Geometry: final body of the model. Coordinates: model frame, mm. A direction names the side the tool comes from. Give positions to 0.01 mm unless a question says otherwise; leave off trailing zeros. Order: outer loops, then holes, each group sorted by start corner. A loop starts at its lowest first (then second) coordinate and runs counter-clockwise, first axis right, second up. Notation, with made-up numbers: M 30,35.5 L 87,35.5 A29 ccw 87,73.5 Z; hole C -13.5,29.25 d5. An arc over 180 degrees is marked long. Use CSV: the item, a comma, the result in double quotes.
```python
from build123d import *

# Parameters (mm, degrees)
SKETCH1_W           = 63.5
SKETCH1_H           = 19.05
BOSS_EXTRUDE1_DEPTH = 6.35
SKETCH2_R           = 2.0955
CUT_EXTRUDE1_DEPTH  = 34.750712955
SKETCH3_W           = 12.7
SKETCH3_H           = 6.35
CUT_EXTRUDE2_DEPTH  = 34.750712955
SKETCH4_W           = 47.625
SKETCH4_H           = 19.05
BOSS_EXTRUDE2_DEPTH = 6.35
SKETCH5_R           = 1.5875
CUT_EXTRUDE3_DEPTH  = 44.184668865
SKETCH6_R           = 1.5875
CUT_EXTRUDE4_DEPTH  = 44.184668865
FILLET3_R           = 6.35
FILLET4_R           = 2.54


with BuildPart() as part:
    # Sketch1 → Boss-Extrude1 (new body)
    with BuildSketch(Plane.XY):
        Rectangle(SKETCH1_W, SKETCH1_H)
    extrude(amount=BOSS_EXTRUDE1_DEPTH)

    # Sketch2 → Cut-Extrude1 (cut, through all)
    with BuildSketch(Plane.XY.offset(6.35)):
        Circle(SKETCH2_R)
    extrude(amount=-CUT_EXTRUDE1_DEPTH, mode=Mode.SUBTRACT)

    # Sketch3 → Cut-Extrude2 (cut, through all)
    with BuildSketch(Plane.XY.offset(6.35)):
        with Locations((-19.05, 0)):
            Rectangle(SKETCH3_W, SKETCH3_H)
    cut_extrude2 = extrude(amount=-CUT_EXTRUDE2_DEPTH, mode=Mode.SUBTRACT)

    # Mirror1: Cut-Extrude2 across plane
    add(cut_extrude2.mirror(Plane(origin=(0, 0, 0), x_dir=(0, 0, 1), z_dir=(1, 0, 0))), mode=Mode.SUBTRACT)

    # Sketch4 → Boss-Extrude2 (add)
    with BuildSketch(Plane.XY.offset(6.35)):
        with Locations((0, 19.05)):
            Rectangle(SKETCH4_W, SKETCH4_H)
    extrude(amount=-BOSS_EXTRUDE2_DEPTH)

    # Sketch5 → Cut-Extrude3 (cut, through all)
    with BuildSketch(Plane.XY.offset(6.35)):
        with Locations((-18.288, 19.05)):
            Circle(SKETCH5_R)
    cut_extrude3 = extrude(amount=-CUT_EXTRUDE3_DEPTH, mode=Mode.SUBTRACT)

    # Mirror2: Cut-Extrude3 across plane
    add(cut_extrude3.mirror(Plane(origin=(0, 0, 0), x_dir=(0, 0, 1), z_dir=(1, 0, 0))), mode=Mode.SUBTRACT)

    # Sketch6 → Cut-Extrude4 (cut, through all)
    with BuildSketch(Plane.XY.offset(6.35)):
        with Locations((0, 6.35)):
            Circle(SKETCH6_R)
    extrude(amount=-CUT_EXTRUDE4_DEPTH, mode=Mode.SUBTRACT)

    # Fillet3
    fillet3_edges = [part.edges().sort_by_distance(p)[0] for p in [
        (23.8125, 28.575, 3.175),
        (-23.8125, 28.575, 3.175),
        (31.75, -9.525, 3.175),
        (-31.75, -9.525, 3.175),
        (-31.75, 9.525, 3.175),
        (31.75, 9.525, 3.175),
    ]]
    fillet(fillet3_edges, radius=FILLET3_R)

    # Fillet4
    fillet4_edges = [part.edges().sort_by_distance(p)[0] for p in [
        (23.8125, 9.525, 3.175),
        (-23.8125, 9.525, 3.175),
    ]]
    fillet(fillet4_edges, radius=FILLET4_R)


solid = part.part
```
1. Section D-D, the plane y = 6.35. Return the cut outline in (x, z).
Answer:
outline,"M -30.9,0 L -1.59,0 L -1.59,6.35 L -30.9,6.35 Z; M 1.59,0 L 30.9,0 L 30.9,6.35 L 1.59,6.35 Z"
2. Pull-direction query (Y, two-part tool) for faces 1 (the face through (0, 28.575, 3)), 2 (the face through (-12.7, 0, 3)), 3 (the face through (0, 10, 6.35)); classes: +Y half, -Y half, draft (parallel to the pull), parting line (faces both ways), or undercut.
Answer:
face 1,"+Y half"
face 2,"undercut"
face 3,"draft"
3. Section A-A, the plane y = 0. Return the cut outline in (x, z), plus the area to 3 significant figures.
Answer:
outline,"M -31.75,0 L -25.4,0 L -25.4,6.35 L -31.75,6.35 Z; M -12.7,0 L -2.1,0 L -2.1,6.35 L -12.7,6.35 Z; M 2.1,0 L 12.7,0 L 12.7,6.35 L 2.1,6.35 Z; M 25.4,0 L 31.75,0 L 31.75,6.35 L 25.4,6.35 Z"
area,"215 mm2"
4. Reachability of faces 4 (the face through (0, -9.525, 3)), 5 (the face through (-23.812, 17, 3)), 6 (the face through (19, 3.175, 3)) from +Z, -Z, +X, -X, +Y, -Y: full face, straight path, thin tool, end or side. Return the list, or none.
Answer:
face 4,"+Z, -Z, +X, -X, -Y"
face 5,"+Z, -Z, -X, +Y"
face 6,"+Z, -Z"
5. Pin query (flat end, axial travel): pin 1 Ø1.9 at (x, y) = (18.288, 19.05) entering from -Z; pin 2 Ø12 at (x, y) = (-0.5, 1.5) entering from -Z; pin 3 Ø1 at (y, z) = (24.5, 4.5) entering from +X; pin 4 Ø3 at (y, z) = (15.5, 2.5) entering from +X. Return the tip coordinate at first contact, or that it passes through.
Answer:
pin 1,"through"
pin 2,"z = 0"
pin 3,"x = 23.56"
pin 4,"x = 23.81"
6. Section B-B, the plane x = 0. Give the number of separate pieces and of enclosed holes in the cut face, plus the area to 3 significant figures.
Answer:
separate pieces,"3"
enclosed holes,"0"
area,"195 mm2"
7. Line query: line 1 (Y direction, x = 0, z = 4) (1 decimal); line 2 (Y direction, x = -18, z = 2) (3 decimals); line 3 (X direction, y = 18.5, z = 2). Output: solid intervals per line, ascending.
Answer:
line 1,"-9.5 to -2.1, 2.1 to 4.8, 7.9 to 28.6"
line 2,"-9.525 to -3.175, 3.175 to 17.489, 20.611 to 28.552"
line 3,"-23.81 to -19.78, -16.8 to 16.8, 19.78 to 23.81"
8. Section C-C, the plane y = 19.05. Return the cut outline in (x, z), plus the area to 3 significant figures.
Answer:
outline,"M -23.81,0 L -19.88,0 L -19.88,6.35 L -23.81,6.35 Z; M -16.7,0 L 16.7,0 L 16.7,6.35 L -16.7,6.35 Z; M 19.88,0 L 23.81,0 L 23.81,6.35 L 19.88,6.35 Z"
area,"262 mm2"
